from build123d import *

# Parameters (mm, degrees)
HEXAGON_DEPTH = 20
HEXAGON_DRAFT = -20.000000000000043
BASE_DEPTH    = 10
SMALL_DEPTH   = 75
FILLET_2_R    = 3
ARRAY_START   = -102.451905284
ARRAY_DEPTH   = 204.903810568
ARRAY_2_DEPTH = 204.903810568
ARRAY_START_2 = 45.459553514
ARRAY_3_DEPTH = 29.540446486
FILLET2_R     = 2
CROQUIS4_W    = 26.916537621276092
CROQUIS4_H    = 24.058782859612524
CROQUIS4_W_2  = 36.99619518821565
CROQUIS4_H_2  = 32.17850701075816
TRIM_DEPTH    = 179.30560151606045


# Read off the part's stored shape, not the designer's step: array
with BuildPart() as part:
    # Croquis1 → hexagon (with draft: the straight prism first)
    with BuildSketch(Plane(origin=(0, 0, 0), x_dir=(1, 0, 0), z_dir=(0, 1, 0))):
        Polygon((46.18802153516988, 0), (23.09401076758485, 39.9999999999999), (-23.09401076758513, 39.99999999999974), (-46.18802153516988, -3.2253e-13), (-23.09401076758457, -40.00000000000006), (23.09401076758541, -39.99999999999958), align=None)
    extrude(amount=HEXAGON_DEPTH)
    # hexagon: the draft: its side faces are tilted about the plane it starts from
    hexagon_sides = [part.faces().sort_by_distance(p)[0] for p in [
        (34.641016151, 10, -20),
        (0, 10, -40),
        (-34.641016151, 10, -20),
        (-34.641016151, 10, 20),
        (0, 10, 40),
        (34.641016151, 10, 20),
    ]]
    draft(hexagon_sides, Plane(origin=(0, 0, 0), x_dir=(1, 0, 0), z_dir=(0, 1, 0)), HEXAGON_DRAFT)

    # Croquis2 → base (add)
    with BuildSketch(Plane(origin=(0, 20, 0), x_dir=(1, 0, 0), z_dir=(0, 1, 0))):
        Polygon((74.99999999999999, -74.99999999999999), (-75.00000000000001, -75.00000000000001), (-75.00000000000001, 74.99999999999999), (74.99999999999999, 75.00000000000001), align=None)
    extrude(amount=BASE_DEPTH)

    # Croquis3 → small (add, through all)
    with BuildSketch(Plane.XY):
        Polygon((-5.773502691896257, 20), (-2.886751345948127, 15), (2.886751345948127, 15), (5.7735026918962555, 20), (2.8867513459481215, 25.000000000000007), (-2.8867513459481278, 25.000000000000007), align=None)
    extrude(amount=-SMALL_DEPTH)

    # fillet 2
    fillet_2_edges = [part.edges().sort_by_distance(p)[0] for p in [
        (4.2277e-13, 0, 39.99999999999982),
        (-34.64101615137723, 0, 20.000000000000206),
        (-34.641016151377514, 0, -19.9999999999997),
        (-1.4921e-13, 0, -39.999999999999815),
        (34.641016151377364, 0, -19.999999999999957),
        (34.64101615137765, 0, 19.999999999999787),
    ]]
    fillet(fillet_2_edges, radius=FILLET_2_R)

    # array outline → array (add)
    with BuildSketch(Plane(origin=(0, 0, 0), x_dir=(0.500000000000004, 0, -0.8660254037844363), z_dir=(0.8660254037844363, 0, 0.5000000000000042)).offset(ARRAY_START)):
        Polygon((-5.773502692, 20), (-2.886751346, 15), (2.886751346, 15), (5.773502692, 20), (2.886751346, 25), (-2.886751346, 25), align=None)
    extrude(amount=ARRAY_DEPTH)

    # array 2 outline → array 2 (add)
    with BuildSketch(Plane(origin=(0, 0, 0), x_dir=(0.49999999999999767, 0, 0.86602540378444), z_dir=(0.8660254037844399, 0, -0.49999999999999795)).offset(ARRAY_START)):
        Polygon((5.773502692, -20), (2.886751346, -15), (-2.886751346, -15), (-5.773502692, -20), (-2.886751346, -25), (2.886751346, -25), align=None)
    extrude(amount=ARRAY_2_DEPTH)

    # array 3 outline → array 3 (add)
    with BuildSketch(Plane.XY.offset(ARRAY_START_2)):
        Polygon((-5.773502692, 20), (-2.886751346, 15), (2.886751346, 15), (5.773502692, 20), align=None)
    extrude(amount=ARRAY_3_DEPTH)

    # fillet2
    fillet2_edges = [part.edges().sort_by_distance(p)[0] for p in [
        (-2.886751346, 15, 60.229776756999996),
        (62.604164741938675, 15, -39.477864699543005),
        (65.49091608793843, 15, 34.47786469945364),
        (-62.60416474193839, 15, -39.477864699543446),
        (2.886751346, 15, 60.229776756999996),
        (-62.60416474193865, 15, 39.47786469954298),
        (-65.49091608793839, 15, -34.47786469945361),
        (2.886751345948127, 15, -60.22977675699644),
        (-2.886751345948127, 15, -60.22977675699643),
        (62.60416474193845, 15, 39.47786469954348),
        (65.49091608793866, 15, -34.47786469945315),
        (-65.49091608793867, 15, 34.47786469945314),
    ]]
    fillet(fillet2_edges, radius=FILLET2_R)

    # Croquis4 → trim (cut, through all)
    with BuildSketch(Plane(origin=(-1.388e-14, 0, -75), x_dir=(-1, 0, 1.9e-16), z_dir=(-1.9e-16, 0, -1))):
        with Locations((-88.45826881063805, 17.97060857019374)):
            Rectangle(CROQUIS4_W, CROQUIS4_H)
        with Locations((93.49809759410783, 13.910746494620925)):
            Rectangle(CROQUIS4_W_2, CROQUIS4_H_2)
    extrude(amount=-TRIM_DEPTH, mode=Mode.SUBTRACT)


solid = part.part
For this review, take the finished solid that the model builds, in its own axes (mm). A direction names the side the tool comes from. Give positions to 0.01 mm unless a question says otherwise; leave off trailing zeros. Write each loop counter-clockwise with the first axis right and the second up, starting at its lowest first coordinate (ties: lowest second). Pieces come first, ordered by that corner, then holes. Notation, with made-up numbers: (56, 21.25) -> (83, 21.25) arc R27 ccw to (83, 59.25) -> close; hole circle Ø8 at (37.5, 70). An arc over 180 degrees is marked (long way). Use CSV: the item, a comma, the result in double quotes.
Q1. Tool access review of faces 5 (the face through (-57.881, 15.275, -30.248)), 6 (the face through (-58, 15, -33)), 7 (the face through (41, 20, -57)), 8 (the face through (56.95, 15.26, 36.02)), 9 (the face through (-58, 15, 33)): name each direction out of +Z, -Z, +X, -X, +Y, -Y from which nothing blocks a thin tool from reaching the whole face with its end or side.
Conclusion:
face 5,"-X, -Y"
face 6,"-Z, -X, -Y"
face 7,"-Z, -Y"
face 8,"+Z, -Y"
face 9,"+Z, -X, -Y"
Q2. Take a section at B-B, the plane y = 3.75. Write out the cut boundary in (x, z).
Conclusion:
outline,"(-47.76, 0) -> (-23.88, -41.36) -> (23.88, -41.36) -> (47.76, 0) -> (23.88, 41.36) -> (-23.88, 41.36) -> close"
Q3. For P1, Ø14, axis at x = 32, z = -60, coming from the -Y side; P2, Ø19.5, axis at x = 47.5, z = -31, coming from the -Y side; P3, Ø8, axis at x = 45.5, y = 6, coming from the -Z side; P4, Ø8, axis at x = -26, z = 34.5, coming from the -Y side, all flat-tipped, find the tip position at first contact; note any pin that passes through.
Conclusion:
P1,"y = 20"
P2,"y = 15"
P3,"z = -13.07"
P4,"y = 0"
Q4. Take a section at A-A, the plane z = -59.5. Write out the cut boundary in (x, y), then the cut area to 3 significant figures.
Conclusion:
outline,"(-75, 20) -> (-5.77, 20) -> (-3.46, 16) arc R2 ccw to (-1.73, 15) -> (1.73, 15) arc R2 ccw to (3.46, 16) -> (5.77, 20) -> (75, 20) -> (75, 30) -> (-75, 30) -> close"
area,"1,540 mm2"
Q5. Mouldability with a two-part tool opening along Z and no side actions: class faces 1 (the face through (58.35, 15.26, -30.55)), 2 (the face through (34.17, 0.56, -20.11)), 3 (the face through (-0.382, 10.861, 43.953)), 4 (the face through (-63, 20, -1)) as pulls with the +Z half, pulls with the -Z half, needs draft (parallel to the pull), parting line crosses it, or undercut.
Conclusion:
face 1,"undercut"
face 2,"pulls with the -Z half"
face 3,"pulls with the +Z half"
face 4,"undercut"
Q6. To check wall thickness, follow probe 1 along X at (y, z) = (17.5, 39); probe 2 along Y at (x, z) = (-60, -0.5); probe 3 along X at (y, z) = (3, -25). State the ranges of each line that lie inside material, in increasing order. Write a range as [from, to].
Conclusion:
probe 1,"[-75, -58.89], [-31.03, 31.03], [58.89, 75]"
probe 2,"[20, 30]"
probe 3,"[-33.02, 33.02]"
